Build history of the part. All positions in model axes, mm. Give positions to 0.01 mm unless a question says otherwise; leave off trailing zeros. Order: outer loops, then holes, each group sorted by start corner. A loop starts at its lowest first (then second) coordinate and runs counter-clockwise, first axis right, second up. Notation, with made-up numbers: (40, 31.25) - (92, 31.25) arc R22 ccw to (92, 62.25) - close; hole circle Ø1 at (81.5, 36). An arc over 180 degrees is marked (long way). Use a Markdown table: item, result. Add a question column.
(1) Slice it at A-A (z = -0.35). Write the cut outline in (x, y).
(2) Slice it at B-B (y = -3.75). Count the separate pieces of the cut face and the enclosed holes in it, then the cut area to 3 significant figures.
(3) Flat gauge pin, fed straight in: pin 1 (4 mm diameter, centred on x = -11.29, y = -2.37, fed in from -Z). Where does the tip first touch, or does it go through?
(4) Wall check: line 1 (X direction, y = -1.25, z = 0.3); line 2 (X direction, y = 4, z = 0.85); line 3 (X direction, y = 0.5, z = -0.1). Give the ranges that are in metal, low to high.
from build123d import *

# Parameters (mm, degrees)
BOSS_EXTRUDE1_DEPTH      = 0.889
BOSS_EXTRUDE1_DEPTH_BACK = 0.889
SKETCH4_W                = 101.6
SKETCH4_H                = 15.875
SKETCH5_R                = 2.2479
CUT_EXTRUDE1_DEPTH       = 52.424062726
SKETCH6_R                = 4.2164
CUT_EXTRUDE2_DEPTH       = 52.447110611
CUT_EXTRUDE2_TAPER       = 49
FILLET1_R                = 0.762


# Read off the part's stored shape, not the designer's step: Sketch-Pattern1
with BuildPart() as part:
    # Sketch4 → Boss-Extrude1 (new, two sides: drawn at the far end of the back side and taken through both)
    with BuildSketch(Plane.XY.offset(-BOSS_EXTRUDE1_DEPTH_BACK)):
        Rectangle(SKETCH4_W, SKETCH4_H)
    extrude(amount=BOSS_EXTRUDE1_DEPTH + BOSS_EXTRUDE1_DEPTH_BACK)

    # Sketch5 → Cut-Extrude1 (cut, symmetric)
    with BuildSketch(Plane.XY):
        with Locations((-33.8582, 2.3749)):
            Circle(SKETCH5_R)
    extrude(amount=CUT_EXTRUDE1_DEPTH, both=True, mode=Mode.SUBTRACT)

    # Sketch6 → Cut-Extrude2 (cut, through all)
    with BuildSketch(Plane.XY.offset(-0.889)):
        with Locations((-33.8582, 2.3749)):
            Circle(SKETCH6_R)
    extrude(amount=CUT_EXTRUDE2_DEPTH, taper=CUT_EXTRUDE2_TAPER, mode=Mode.SUBTRACT)

    # Sketch-Pattern1 outline → Sketch-Pattern1 (revolve, cut)
    with BuildSketch(Plane(origin=(11.286066667, 2.3749, 0), x_dir=(1, 0, 0), z_dir=(0, -1, 0))):
        Polygon((0, -0.889), (4.2164, -0.889), (2.2479, 0.822190943), (2.2479, 0.889), (0, 0.889), align=None)
    revolve(axis=Axis((11.286066667, 2.3749, 0), (0, 0, 1)), mode=Mode.SUBTRACT)

    # Sketch-Pattern1 2 outline → Sketch-Pattern1 2 (revolve, cut)
    with BuildSketch(Plane(origin=(33.8582, -2.3749, 0), x_dir=(1, 0, 0), z_dir=(0, -1, 0))):
        Polygon((0, -0.889), (4.2164, -0.889), (2.2479, 0.822190943), (2.2479, 0.889), (0, 0.889), align=None)
    revolve(axis=Axis((33.8582, -2.3749, 0), (0, 0, 1)), mode=Mode.SUBTRACT)

    # Sketch-Pattern1 3 outline → Sketch-Pattern1 3 (revolve, cut)
    with BuildSketch(Plane(origin=(-11.286066667, -2.3749, 0), x_dir=(1, 0, 0), z_dir=(0, -1, 0))):
        Polygon((0, -0.889), (4.2164, -0.889), (2.2479, 0.822190943), (2.2479, 0.889), (0, 0.889), align=None)
    revolve(axis=Axis((-11.286066667, -2.3749, 0), (0, 0, 1)), mode=Mode.SUBTRACT)

    # Fillet1
    fillet1_edges = [part.edges().sort_by_distance(p)[0] for p in [
        (-50.8, 7.9375, 0),
        (50.8, 7.9375, 0),
        (50.8, -7.9375, 0),
        (-50.8, -7.9375, 0),
    ]]
    fillet(fillet1_edges, radius=FILLET1_R)


solid = part.part
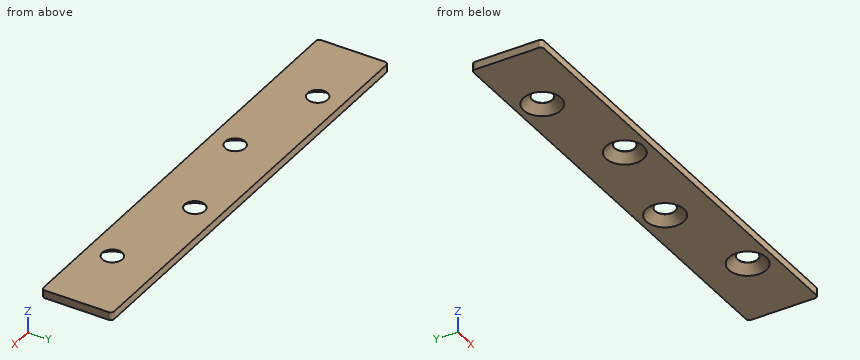
Solution:
| question | item | result |
|---|---|---|
| 1 | outline | (-50.8, -7.18) arc R0.76 ccw to (-50.04, -7.94) - (50.04, -7.94) arc R0.76 ccw to (50.8, -7.18) - (50.8, 7.18) arc R0.76 ccw to (50.04, 7.94) - (-50.04, 7.94) arc R0.76 ccw to (-50.8, 7.18) - close; hole circle Ø7.19 at (-33.86, 2.37); hole circle Ø7.19 at (-11.29, -2.37); hole circle Ø7.19 at (11.29, 2.37); hole circle Ø7.19 at (33.86, -2.37) |
| 2 | separate pieces | 3 |
| 2 | enclosed holes | 0 |
| 2 | area | 160 mm2 |
| 3 | pin 1 | through |
| 4 | line 1 | -50.8 to -13.9, -8.67 to 31.24, 36.48 to 50.8 |
| 4 | line 2 | -50.8 to -35.41, -32.31 to 9.73, 12.84 to 50.8 |
| 4 | line 3 | -50.8 to -36.58, -31.13 to -12.92, -9.65 to 8.56, 14.01 to 32.22, 35.5 to 50.8 |
